Input: part model. Units: mm. Frame: model coordinates. A direction names the side the tool comes from. Round coordinates to 2 decimals unless told otherwise and drop trailing zeros. Write each loop counter-clockwise with the first axis right and the second up, starting at its lowest first coordinate (ties: lowest second). Pieces come first, ordered by that corner, then holes. Notation, with made-up numbers: (-16, 22.25) -> (2, 22.25) arc R23 ccw to (2, 50.25) -> close; hole circle Ø4 at (-1, -31.5). An arc over 180 degrees is marked (long way). Write item = value, one per line.
```python
from build123d import *

# Parameters (mm, degrees)
BOSS_EXTRUDE1_DEPTH = 61.2
SKETCH3_R           = 1.95
CUT_EXTRUDE1_DEPTH  = 2


with BuildPart() as part:
    # Sketch2 → Boss-Extrude1 (new body)
    with BuildSketch(Plane(origin=(0, 0, 0), x_dir=(0, 0, -1), z_dir=(1, 0, 0))):
        with BuildLine():
            Line((0, 0), (-10, 0))
            Line((-10, 0), (-10, 7.898424126))
            Line((-10, 7.898424126), (-16.749767181, 13.862964902))
            ThreePointArc((-16.749767181, 13.862964902), (-29, 18.5), (-41.250232819, 13.862964902))
            Line((-41.250232819, 13.862964902), (-48, 7.898424126))
            Line((-48, 7.898424126), (-48, 0))
            Line((-48, 0), (-60, 0))
            Line((-60, 0), (-60, 6.817623549))
            Line((-60, 6.817623549), (-66.59398274, 11.918310368))
            ThreePointArc((-66.59398274, 11.918310368), (-76.2, 15.2), (-85.80601726, 11.918310368))
            Line((-85.80601726, 11.918310368), (-92.4, 6.817623549))
            Line((-92.4, 6.817623549), (-92.4, 0))
            Line((-92.4, 0), (-102.4, 0))
            Line((-102.4, 0), (-102.4, 2))
            Line((-102.4, 2), (-94.4, 2))
            Line((-94.4, 2), (-94.4, 7.799074738))
            Line((-94.4, 7.799074738), (-87.029713726, 13.500260734))
            ThreePointArc((-87.029713726, 13.500260734), (-76.2, 17.2), (-65.370286274, 13.500260734))
            Line((-65.370286274, 13.500260734), (-58, 7.799074738))
            Line((-58, 7.799074738), (-58, 2))
            Line((-58, 2), (-50, 2))
            Line((-50, 2), (-50, 8.800073553))
            Line((-50, 8.800073553), (-42.574582313, 15.361663811))
            ThreePointArc((-42.574582313, 15.361663811), (-29, 20.5), (-15.425417687, 15.361663811))
            Line((-15.425417687, 15.361663811), (-8, 8.800073553))
            Line((-8, 8.800073553), (-8, 2))
            Line((-8, 2), (0, 2))
            Line((0, 2), (0, 0))
        make_face()
    extrude(amount=BOSS_EXTRUDE1_DEPTH)

    # Sketch3 → Cut-Extrude1 (cut)
    with BuildSketch(Plane(origin=(0, 2, 0), x_dir=(1, 0, 0), z_dir=(0, 1, 0))):
        with Locations(Location((12.24, -3.93, 0), (0, 0, 270))):
            Circle(SKETCH3_R)
        with Locations(Location((24.48, -3.93, 0), (0, 0, 270))):
            Circle(SKETCH3_R)
        with Locations(Location((36.72, -3.93, 0), (0, 0, 270))):
            Circle(SKETCH3_R)
        with Locations(Location((48.96, -3.93, 0), (0, 0, 270))):
            Circle(SKETCH3_R)
        with Locations(Location((12.24, -53.992271577, 0), (0, 0, 270))):
            Circle(SKETCH3_R)
        with Locations(Location((24.48, -53.992271577, 0), (0, 0, 270))):
            Circle(SKETCH3_R)
        with Locations(Location((36.72, -53.992271577, 0), (0, 0, 270))):
            Circle(SKETCH3_R)
        with Locations(Location((48.96, -53.992271577, 0), (0, 0, 270))):
            Circle(SKETCH3_R)
        with Locations(Location((12.24, -98.47, 0), (0, 0, 270))):
            Circle(SKETCH3_R)
        with Locations(Location((24.48, -98.47, 0), (0, 0, 270))):
            Circle(SKETCH3_R)
        with Locations(Location((36.72, -98.47, 0), (0, 0, 270))):
            Circle(SKETCH3_R)
        with Locations(Location((48.96, -98.47, 0), (0, 0, 270))):
            Circle(SKETCH3_R)
    extrude(amount=-CUT_EXTRUDE1_DEPTH, mode=Mode.SUBTRACT)


solid = part.part
```
1) Draft query along Z for faces 1 (the face through (38.038, 1.014, 52.555)), 2 (the face through (30, 4, 48)), 3 (the face through (30, 0, 97)), 4 (the face through (30, 5, 94.4)). Return one class per face: +Z half, -Z half, draft (parallel to the pull), parting line (faces both ways), or undercut.
Solutions:
face_1 = undercut
face_2 = undercut
face_3 = draft
face_4 = +Z half
2) Cut plane C-C (z = 51). Return the cut outline in (x, y), and give its area (3 significant figures).
Solutions:
outline = (0, 0) -> (61.2, 0) -> (61.2, 2) -> (0, 2) -> close
area = 122 mm^2
3) First-contact query: P1, Ø1.5, axis at x = 30.5, y = 8.5, coming from the +Z side; P2, Ø6, axis at x = 24.48, z = 98.47, coming from the -Y side; P3, Ø2, axis at x = 22.5, z = 31, coming from the -Y side; P4, Ø2.5, axis at x = 31, z = 55.5, coming from the +Y side. Flat tips, straight axial feed; report the tip coordinate or a pass-through.
Solutions:
P1 = 94.4
P2 = 0
P3 = 18.26
P4 = 2
4) Access query for faces 5 (the face through (30, 2, 54)), 6 (the face through (30, 3, 92.4)), 7 (the face through (26.124, 1.014, 99.518)). Directions: +Z, -Z, +X, -X, +Y, -Y. A direction counts if a zero-diameter tool reaches every point of the face in a straight line with its end or side. Return the directions, or none.
Solutions:
face_5 = +X, -X, +Y
face_6 = +X, -X, -Y
face_7 = +Y, -Y
5) Line query: L1, parallel to Z at x = 48, y = 3.75; L2, parallel to X at y = 1.2, z = 3.93; L3, parallel to Z at x = 46.5, y = 1. Output: solid intervals per line, ascending. Write a range as from..to.
Solutions:
L1 = 8..10, 48..50, 58..60, 92.4..94.4
L2 = 0..10.29, 14.19..22.53, 26.43..34.77, 38.67..47.01, 50.91..61.2
L3 = 0..10, 48..60, 92.4..102.4
6) Cut plane D-D (z = 81). Return the cut outline in (x, y), and give its area (3 significant figures).
Solutions:
outline = (0, 14.45) -> (61.2, 14.45) -> (61.2, 16.54) -> (0, 16.54) -> close
area = 128 mm^2
7) Cut plane A-A (z = 3.93). Return the cut outline in (x, y).
Solutions:
outline = (0, 0) -> (10.29, 0) -> (10.29, 2) -> (0, 2) -> close; (14.19, 0) -> (22.53, 0) -> (22.53, 2) -> (14.19, 2) -> close; (26.43, 0) -> (34.77, 0) -> (34.77, 2) -> (26.43, 2) -> close; (38.67, 0) -> (47.01, 0) -> (47.01, 2) -> (38.67, 2) -> close; (50.91, 0) -> (61.2, 0) -> (61.2, 2) -> (50.91, 2) -> close
8) Cut plane B-B (x = 36.72). Count the separate pieces of the cut face and the enclosed holes in it, and give its area (3 significant figures).
Solutions:
separate_pieces = 4
enclosed_holes = 0
area = 261 mm^2
